Input: part model. Units: mm. Frame: model coordinates. A direction names the side the tool comes from. Coordinates: 2 decimals unless noted, no trailing zeros. Order: outer loops, then holes, each group sorted by start corner. A loop starts at its lowest first (then second) coordinate and runs counter-clockwise, first axis right, second up. Notation, with made-up numbers: (52.25, 32) -> (83.25, 32) arc R20 cw to (83.25, 42) -> close; hole circle Ø1 at (66, 36.25). An arc over 180 degrees is marked (long way). Use CSV: the item, a comma, the result in double quotes. Start each with the question number.
```python
from build123d import *

# Parameters (mm, degrees)
F0_R      = 30.48
F1_DEPTH  = 5.08
F3_DEPTH  = 5.08
F4_COUNT  = 20
F5_R      = 26.67
F6_DEPTH  = 5.081
F7_DEPTH  = 5.081
F9_DEPTH  = 5.08
F10_COUNT = 3
F11_R     = 3.302
F12_DEPTH = 5.081


with BuildPart() as f1:
    # F0 (on Top) → F1 (new body)
    with BuildSketch(Plane.XY):
        Circle(F0_R)
    extrude(amount=F1_DEPTH)

    # F4: F3 ×20 about axis
    f4_axis = Axis((0, 0, 5.08), (0, 0, 1))


with BuildPart() as f3:
    # F2 (on face) → F3 (new body, through all)
    with BuildSketch(Plane.XY.offset(5.08)):
        with BuildLine():
            Line((-5.7019906833, 29.9389965966), (0.9482987996, 30.4623857298))
            ThreePointArc((0.9482987996, 30.4623857298), (-0.0033837458, 34.8376195512), (-3.0033778465, 38.1615338182))
            ThreePointArc((-3.0033778465, 38.1615338182), (-5.4464622915, 34.4092399792), (-5.7019906833, 29.9389965966))
        make_face()
    extrude(amount=-F3_DEPTH)


with BuildPart() as f1_1:
    add(f1.part)
    for i in range(1, F4_COUNT):
        add(f3.part.rotate(f4_axis, i * 360 / F4_COUNT))

    # F5 (on face) → F6 (cut, through all)
    with BuildSketch(Plane.XY.offset(5.08)):
        Circle(F5_R)
    extrude(amount=-F6_DEPTH, mode=Mode.SUBTRACT)

    # F5 (on face) → F7 (cut, through all)
    with BuildSketch(Plane.XY.offset(5.08)):
        Circle(F5_R)
    extrude(amount=-F7_DEPTH, mode=Mode.SUBTRACT)



with BuildPart() as f9:
    # F8 (on face) → F9 (new body, through all)
    with BuildSketch(Plane.XY.offset(5.08)):
        with BuildLine():
            Line((-4.6311968984, 26.2648227728), (-1.1026659282, 6.2535292316))
            ThreePointArc((-1.1026659282, 6.2535292316), (0, -6.35), (1.1026659282, 6.2535292316))
            Line((1.1026659282, 6.2535292316), (4.6311968984, 26.2648227728))
            ThreePointArc((4.6311968984, 26.2648227728), (0, 26.67), (-4.6311968984, 26.2648227728))
        make_face()
    extrude(amount=-F9_DEPTH)


with BuildPart() as f1_2:
    add(f1_1.part)

    add(f3.part)  # F10 merges F3

    add(f9.part)  # F10 merges F9
    # F10: F9 ×3 about axis
    f10_axis = Axis((0, 0, 5.08), (0, 0, 1))
    for i in range(1, F10_COUNT):
        add(f9.part.rotate(f10_axis, i * 360 / F10_COUNT))

    # F11 (on face) → F12 (cut, through all)
    with BuildSketch(Plane.XY.offset(5.08)):
        Circle(F11_R)
    extrude(amount=-F12_DEPTH, mode=Mode.SUBTRACT)


solid = f1_2.part
```
1. Section B-B on y = 0. Return loops of the section in (x, z), then the cut area to 3 significant figures.
2. Contact query for flat-ended pins moving along their axis: P1, Ø3, axis at y = 19, z = 4.5, coming from the +X side; P2, Ø2, axis at y = -7.5, z = 3, coming from the +X side; P3, Ø5.5, axis at x = 0, y = 0, coming from the +Z side; P4, Ø3, axis at x = -10, z = 4.5, coming from the -Y side. Output: stop coordinate, or through.
3. Section A-A on x = 0. Return loops of the section in (y, z).
4. Section C-C on z = 0.8. State how many separate pieces and enclosed holes the cut face has, then the cut area to 3 significant figures.
5. Pull-direction query (X, two-part tool) for faces 4 (the face through (28.15, 20.42, 2.58)), 5 (the face through (1, -4, 0)), 6 (the face through (-24.65, 24.7, 2.58)), 7 (the face through (-23, 20, 3)); classes: released by +X, released by -X, zero draft, split by the parting line, or undercut.
6. Material intervals for line 1 along Y through (x, z) = (-19.5, 1.35); line 2 along X through (y, z) = (13, 3.35); line 3 along Y through (x, z) = (33, 3), sorted ascending.
7. Access query for faces 1 (the face through (-2.412, -30.384, 2.504)), 2 (the face through (-12.756, -10.704, 2.576)), 3 (the face through (-30.384, 2.412, 2.504)). Directions: +Z, -Z, +X, -X, +Y, -Y. A direction counts if a zero-diameter tool reaches every point of the face in a straight line with its end or side. Return the directions, or none.
Values follow:
1,outline,"(-34.83, 0) -> (-26.67, 0) -> (-26.67, 5.08) -> (-34.83, 5.08) -> close; (-6.35, 0) -> (-3.3, 0) -> (-3.3, 5.08) -> (-6.35, 5.08) -> close; (3.3, 0) -> (6.35, 0) -> (6.35, 5.08) -> (3.3, 5.08) -> close; (26.67, 0) -> (34.83, 0) -> (34.83, 5.08) -> (26.67, 5.08) -> close"
1,area,"114 mm2"
2,P1,"stops at x = 28.19"
2,P2,"stops at x = 37.01"
2,P3,"passes through"
2,P4,"stops at y = -37.22"
3,outline,"(-34.83, 0) -> (-26.67, 0) -> (-26.67, 5.08) -> (-34.83, 5.08) -> close; (-6.35, 0) -> (-3.3, 0) -> (-3.3, 5.08) -> (-6.35, 5.08) -> close; (3.3, 0) -> (34.83, 0) -> (34.83, 5.08) -> (3.3, 5.08) -> close"
4,separate pieces,"1"
4,enclosed holes,"4"
4,area,"1,910 mm2"
5,face 4,"released by +X"
5,face 5,"zero draft"
5,face 6,"released by -X"
5,face 7,"undercut"
6,line 1,"y = -32.57 to -25.33, -23.43 to -18.19, -16.36 to -7.1, 18.19 to 27.6"
6,line 2,"x = -27.61 to -23.29, -2.29 to 2.29, 23.29 to 34.74"
6,line 3,"y = -10.78 to -4.61, -0.69 to 5.78, 10.64 to 15.58"
7,face 1,"+Z, -Z, -Y"
7,face 2,"+Z, -Z"
7,face 3,"+Z, -Z, -X"
